Design review of the part shown in the three views and the two pictorial views. Dimensions are in mm from the part's minimum x, y and z. Round coordinates to 2 decimals unless told otherwise and drop trailing zeros. Order: outer loops, then holes, each group sorted by start corner. A loop starts at its lowest first (then second) coordinate and runs counter-clockwise, first axis right, second up.
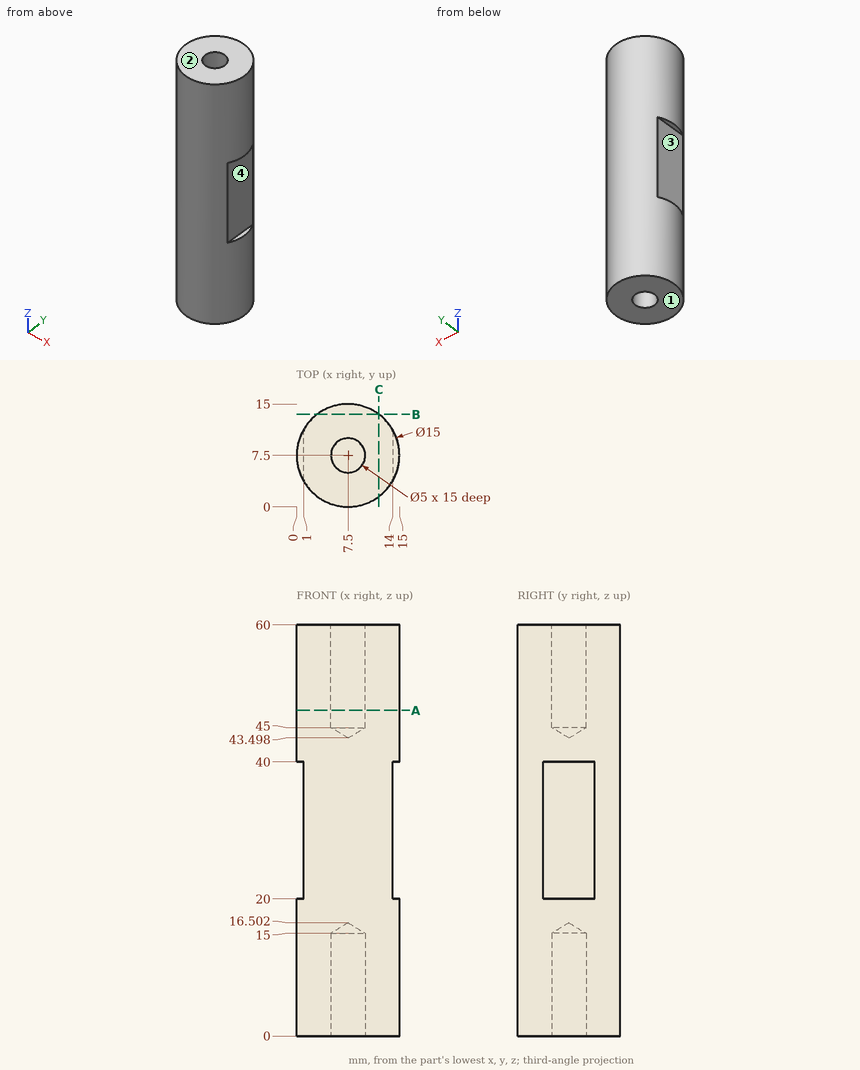
1) To check wall thickness, follow line 1 along X through (y, z) = (7.5, 3.25); line 2 along Z through (x, y) = (14.5, 7.5). State the ranges of each line that lie inside material, in increasing order.
Results:
line 1: x = 0 to 5, 10 to 15
line 2: z = 0 to 20, 40 to 60
2) Take a section at C-C on x = 12. Give the boundary of the cut face in (y, z).
Results:
outline: (1.5, 0) - (13.5, 0) - (13.5, 60) - (1.5, 60) - close
3) Take a section at A-A on z = 47.5. Give the boundary of the cut face in (x, y).
Results:
outline: circle Ø15 at (7.5, 7.5); hole circle Ø5 at (7.5, 7.5)
4) The part is to be moulded in two halves that separate along Z. For the marked faces 1, 2, 3 and 4, say which applies: released by +Z, released by -Z, zero draft, split by the parting line, or undercut.
Results:
face 1: released by -Z
face 2: released by +Z
face 3: undercut
face 4: undercut
5) Clearance check with flat-ended pins moving along their axes: P1, Ø8, axis at y = 9.5, z = 33.5, coming from the -X side; P2, Ø1.1, axis at x = 14.5, y = 6.5, coming from the -Z side; P3, Ø8, axis at y = 9, z = 28, coming from the +X side; P4, Ø2, axis at x = 7.5, y = 8, coming from the +Z side. State where each tip first meets the part, or that it passes through.
Results:
P1: stops at x = 1
P2: stops at z = 0
P3: stops at x = 14
P4: stops at z = 44.4
6) Take a section at B-B on y = 13.5. Give the boundary of the cut face in (x, z).
Results:
outline: (3, 0) - (12, 0) - (12, 60) - (3, 60) - close
